from build123d import *

# Parameters (mm, degrees)
F0_W     = 120
F0_H     = 60
F1_DEPTH = 5
F3_D     = 4.2
F5_D     = 4.3


with BuildPart() as f1:
    # F0 (on Front) → F1 (new body)
    with BuildSketch(Plane.XZ):
        with Locations((60, 30)):
            Rectangle(F0_W, F0_H)
    extrude(amount=F1_DEPTH)

    # F3 (through all)
    with Locations(Plane(origin=(0, 0, 0), x_dir=(1, 0, 0), z_dir=(0, 1, 0))):
        with Locations((10, -40), (10, -20), (110, -20), (110, -40)):
            Hole(F3_D / 2)

    # F5 (through all)
    with Locations(Plane(origin=(0, 0, 0), x_dir=(1, 0, 0), z_dir=(0, 1, 0))):
        with Locations((40, -45), (40, -15), (80, -15), (80, -45)):
            Hole(F5_D / 2)


solid = f1.part
Input: part model. Units: mm. Frame: model coordinates. Give positions to 0.01 mm unless a question says otherwise; leave off trailing zeros. Loops run counter-clockwise (first coordinate to the right, second up) from the corner with the lowest first, then second, coordinate; pieces in that order, holes last. Notation, with made-up numbers: (64.25, 63.25) -> (101.25, 63.25) arc R4 ccw to (101.25, 68.25) -> close; hole circle Ø3 at (35.25, -38). An arc over 180 degrees is marked (long way). Answer as a JSON object with one key per item and string values. Group by question number.
Item 1: Line query: probe 1 along X at (y, z) = (-1.85, 15); probe 2 along Z at (x, y) = (10, -1.35); probe 3 along X at (y, z) = (-1.2, 20). Output: solid intervals per line, ascending.
Item 2: Cut plane B-B, the plane x = 80. Return the cut outline in (y, z).
Item 3: Cut plane C-C, the plane y = -2.75. State how many separate pieces and enclosed holes the cut face has, and give its area (3 significant figures).
Item 4: Cut plane A-A, the plane z = 45. Return the cut outline in (x, y), and give its area (3 significant figures).
Item 5: Pull-direction query (Z, two-part tool) for faces 1 (the flat face through (59, -2, 0)), 2 (the cylindrical face through (38.84, -2.53, 43.19)), 3 (the flat face through (0, -2, 30)); classes: released by +Z, released by -Z, zero draft, split by the parting line, or undercut.
Item 6: Pin query (flat end, axial travel): P1, Ø5, axis at x = 10, z = 20, coming from the -Y side; P2, Ø3.5, axis at x = 10, z = 40, coming from the +Y side (3 decimals). Return the tip coordinate at first contact, or that it passes through.
Checks:
{
 "1": {"probe 1": "x = 0 to 37.85, 42.15 to 77.85, 82.15 to 120", "probe 2": "z = 0 to 17.9, 22.1 to 37.9, 42.1 to 60", "probe 3": "x = 0 to 7.9, 12.1 to 107.9, 112.1 to 120"},
 "2": {"outline": "(-5, 0) -> (0, 0) -> (0, 12.85) -> (-5, 12.85) -> close; (-5, 17.15) -> (0, 17.15) -> (0, 42.85) -> (-5, 42.85) -> close; (-5, 47.15) -> (0, 47.15) -> (0, 60) -> (-5, 60) -> close"},
 "3": {"separate pieces": "1", "enclosed holes": "8", "area": "7,090 mm²"},
 "4": {"outline": "(0, -5) -> (37.85, -5) -> (37.85, 0) -> (0, 0) -> close; (42.15, -5) -> (77.85, -5) -> (77.85, 0) -> (42.15, 0) -> close; (82.15, -5) -> (120, -5) -> (120, 0) -> (82.15, 0) -> close", "area": "557 mm²"},
 "5": {"face 1": "released by -Z", "face 2": "undercut", "face 3": "zero draft"},
 "6": {"P1": "stops at y = -5", "P2": "passes through"}
}
